Source: CAD feature listing. Evaluate the final solid. Frame: model axes, mm. A direction names the side the tool comes from. Round coordinates to 2 decimals unless told otherwise and drop trailing zeros. Order: outer loops, then holes, each group sorted by start corner. A loop starts at its lowest first (then second) coordinate and runs counter-clockwise, first axis right, second up. Notation, with made-up numbers: (10, 82.25) - (32, 82.25) arc R27 ccw to (32, 99.25) - close; hole circle Ø6 at (-39.75, 61.5). An arc over 180 degrees is marked (long way). Return JSON: item names as keys, results as strings. Group by question number.
1) Section A-A, the plane z = -3.75. Return loops of the section in (x, y), plus the area to 3 significant figures.
2) Contact query for flat-ended pins moving along their axis: P1, Ø6, axis at x = 26.5, z = 0, coming from the -Y side; P2, Ø8, axis at x = -15.5, z = 1, coming from the +Y side. Output: stop coordinate, or through.
3) Mould query, pull axis Z, two halves, no side actions, for faces 1 (the flat face through (0, 0, 11)), 2 (the flat face through (0, 1.5, 0)), 3 (the flat face through (0, 3, -11.9)). Classes: pulls with the +Z half, pulls with the -Z half, needs draft (parallel to the pull), parting line crosses it, or undercut.
4) Section B-B, the plane x = -20. Return loops of the section in (y, z), plus the area to 3 significant figures.
5) Ray query, line 1 (Z direction, x = -16.5, y = 0.5); line 2 (Y direction, x = 8, z = -5.5); line 3 (Y direction, x = 8.5, z = -8.25). Return the intervals inside material, ascending. Write a range as from..to.
6) Access query for faces 4 (the flat face through (0, 1, 10.4)), 5 (the flat face through (0, 6.5, 0)), 6 (the flat face through (0, 0, -11)). Directions: +Z, -Z, +X, -X, +Y, -Y. A direction counts if a zero-diameter tool reaches every point of the face in a straight line with its end or side. Return the directions, or none.
```python
from build123d import *

# Parameters (mm, degrees)
CROQUIS1_W              = 70.7
CROQUIS1_H              = 23.8
SALIENTE_EXTRUIR1_DEPTH = 7
CROQUIS2_W              = 64.5
CROQUIS2_H              = 16.4
CORTAR_EXTRUIR1_DEPTH   = 0.5
REDONDEO1_R             = 0.5
CROQUIS3_W              = 0.5
CROQUIS3_H              = 0.5
CORTAR_EXTRUIR2_DEPTH   = 7
CROQUIS4_W              = 70.7
CROQUIS4_H              = 20.8
CORTAR_EXTRUIR3_DEPTH   = 1.5
CROQUIS5_W              = 66.7
CROQUIS5_H              = 1.5
CORTAR_EXTRUIR4_DEPTH   = 1
REDONDEO2_R             = 0.5


with BuildPart() as part:
    # Croquis1 → Saliente-Extruir1 (new body)
    with BuildSketch(Plane(origin=(0, 0, 0), x_dir=(1, 0, 0), z_dir=(0, 1, 0))):
        Rectangle(CROQUIS1_W, CROQUIS1_H)
    extrude(amount=SALIENTE_EXTRUIR1_DEPTH)

    # Croquis2 → Cortar-Extruir1 (cut)
    with BuildSketch(Plane(origin=(0, 7, 0), x_dir=(1, 0, 0), z_dir=(0, 1, 0))):
        Rectangle(CROQUIS2_W, CROQUIS2_H)
    extrude(amount=-CORTAR_EXTRUIR1_DEPTH, mode=Mode.SUBTRACT)

    # Redondeo1
    redondeo1_edges = [part.edges().sort_by_distance(p)[0] for p in [
        (-32.25, 6.75, 8.2),
        (-32.25, 6.75, -8.2),
        (32.25, 6.75, -8.2),
        (32.25, 6.75, 8.2),
    ]]
    fillet(redondeo1_edges, radius=REDONDEO1_R)

    # Croquis3 → Cortar-Extruir2 (cut)
    with BuildSketch(Plane(origin=(0, 7, 0), x_dir=(1, 0, 0), z_dir=(0, 1, 0))):
        with Locations((-35.1, 11.65)):
            Rectangle(CROQUIS3_W, CROQUIS3_H)
        with Locations((-35.1, -11.65)):
            Rectangle(CROQUIS3_W, CROQUIS3_H)
        with Locations((35.1, -11.65)):
            Rectangle(CROQUIS3_W, CROQUIS3_H)
        with Locations((35.1, 11.65)):
            Rectangle(CROQUIS3_W, CROQUIS3_H)
    extrude(amount=-CORTAR_EXTRUIR2_DEPTH, mode=Mode.SUBTRACT)

    # Croquis4 → Cortar-Extruir3 (cut)
    with BuildSketch(Plane.XZ):
        Rectangle(CROQUIS4_W, CROQUIS4_H)
    extrude(amount=-CORTAR_EXTRUIR3_DEPTH, mode=Mode.SUBTRACT)

    # Croquis5 → Cortar-Extruir4 (cut)
    with BuildSketch(Plane(origin=(0, 7, 0), x_dir=(1, 0, 0), z_dir=(0, 1, 0))):
        with Locations((0, 10.15)):
            Rectangle(CROQUIS5_W, CROQUIS5_H)
        with Locations((0, -10.15)):
            Rectangle(CROQUIS5_W, CROQUIS5_H)
    extrude(amount=-CORTAR_EXTRUIR4_DEPTH, mode=Mode.SUBTRACT)

    # Redondeo2
    redondeo2_edges = [part.edges().sort_by_distance(p)[0] for p in [
        (0, 6, -10.9),
        (0, 6, -9.4),
        (0, 6, 9.4),
        (0, 6, 10.9),
    ]]
    fillet(redondeo2_edges, radius=REDONDEO2_R)


solid = part.part
```
Geometry check:
{
 "1": {"outline": "(-35.35, 1.5) - (35.35, 1.5) - (35.35, 7) - (32.25, 7) - (32.25, 6.5) - (-32.25, 6.5) - (-32.25, 7) - (-35.35, 7) - close", "area": "357 mm2"},
 "2": {"P1": "y = 1.5", "P2": "y = 6.5"},
 "3": {"face 1": "needs draft", "face 2": "undercut", "face 3": "pulls with the -Z half"},
 "4": {"outline": "(0, -11.9) - (7, -11.9) - (7, -10.9) - (6.5, -10.9) arc R0.5 cw to (6, -10.4) - (6, -9.9) arc R0.5 cw to (6.5, -9.4) - (7, -9.4) - (7, -8.2) - (6.5, -8.2) - (6.5, 8.2) - (7, 8.2) - (7, 9.4) - (6.5, 9.4) arc R0.5 cw to (6, 9.9) - (6, 10.4) arc R0.5 cw to (6.5, 10.9) - (7, 10.9) - (7, 11.9) - (0, 11.9) - (0, 10.4) - (1.5, 10.4) - (1.5, -10.4) - (0, -10.4) - close", "area": "124 mm2"},
 "5": {"line 1": "-11.9..-10.4, 10.4..11.9", "line 2": "1.5..6.5", "line 3": "1.5..7"},
 "6": {"face 4": "+X, -X, -Y", "face 5": "+Y", "face 6": "+Z, -Z, +X, -X, -Y"}
}
